Autodesk Inventor part; units mm, degrees
ref_plane "YZ Plane" through (0, 0, 0) normal (1, 0, 0) x (0, 1, 0)
ref_plane "XZ Plane" through (0, 0, 0) normal (0, 1, 0) x (-1, 0, 0)
ref_plane "XY Plane" through (0, 0, 0) normal (0, 0, 1) x (1, 0, 0)
sketch "Sketch2" plane through (0, 0, 1) normal (0, 0, 1) x (1, 0, 0)
  line L0 (-38.5, 36) -> (38.5, 36)
  line L1 (-48.5, 26) -> (-38.5, 26)
  line L2 (-38.5, 26) -> (-38.5, 36)
  line L3 (-38.5, 36) -> (-48.5, 36)
  line L4 (-48.5, 36) -> (-48.5, 26)
  line L5 (-48.5, 26) -> (-38.5, 36) construction
  line L6 (-38.5, 26) -> (-48.5, 36) construction
  line L7 (0, 0) -> (0, 7.0571)
  line L8 (0, 0) -> (6.6312, 0)
  line L9 (-38.5, -36) -> (-38.5, 36)
  line L10 (48.5, 26) -> (38.5, 26)
  line L11 (38.5, 26) -> (38.5, 36)
  line L12 (38.5, 36) -> (48.5, 36)
  line L13 (48.5, 36) -> (48.5, 26)
  line L14 (48.5, 26) -> (38.5, 36) construction
  line L15 (38.5, 26) -> (48.5, 36) construction
  circle A0 centre (-44.5, 31) radius 1.6
  circle A1 centre (44.5, 31) radius 1.6
  line L16 (38.5, -36) -> (-38.5, -36)
  line L17 (-5, -46) -> (5, -46)
  line L18 (5, -46) -> (5, -36)
  line L19 (5, -36) -> (-5, -36)
  line L20 (-5, -36) -> (-5, -46)
  line L21 (-5, -46) -> (5, -36) construction
  line L22 (5, -46) -> (-5, -36) construction
  circle A2 centre (0, -42) radius 1.6
  line L23 (-48.5, -26) -> (-38.5, -26)
  line L24 (-38.5, -26) -> (-38.5, -36)
  line L25 (-38.5, -36) -> (-48.5, -36)
  line L26 (-48.5, -36) -> (-48.5, -26)
  line L27 (-48.5, -26) -> (-38.5, -36) construction
  line L28 (-38.5, -26) -> (-48.5, -36) construction
  line L29 (38.5, -26) -> (38.5, -36)
  line L30 (38.5, -36) -> (48.5, -36)
  line L31 (48.5, -36) -> (48.5, -26)
  line L32 (48.5, -26) -> (38.5, -36) construction
  line L33 (38.5, -26) -> (48.5, -36) construction
  line L34 (48.5, -26) -> (38.5, -26)
  circle A3 centre (-44.5, -31) radius 1.6
  circle A4 centre (44.5, -31) radius 1.6
  point P0 (-43.5, 31)
  point P1 (43.5, 31)
  point P2 (0, -41)
  point P3 (-38.5, -36)
  point P4 (-43.5, -31)
  point P5 (43.5, -31)
  dimension "d5" = 10
  dimension "d6" = 10
  dimension "d10" = 3.2
  dimension "d12" = 4
  dimension "d18" = 3.2
  dimension "d19" = 10
  dimension "d20" = 10
  dimension "d21" = 4
  dimension "d22" = 5
sketch "Sketch1" plane through (0, 0, 0) normal (0, 0, 1) x (1, 0, 0)
  line L0 (-38.5, 36) -> (38.5, 36)
  line L1 (38.5, 36) -> (38.5, -36)
  line L2 (38.5, -36) -> (-38.5, -36)
  line L3 (-38.5, -36) -> (-38.5, 36)
  line L4 (-38.5, 36) -> (38.5, -36) construction
  line L5 (38.5, 36) -> (-38.5, -36) construction
  point P0 (0, 0)
  dimension "d0" = 72
  dimension "d1" = 77
extrude "Plate1" add sketch "Sketch1" along normal blind 1
sketch "Sketch3" plane through (0, 0, 1) normal (0, 0, 1) x (1, 0, 0)
  line L0 (-22.5, 27.5) -> (-12.5, 27.5)
  line L1 (-7.5, 22.5) -> (-7.5, 12.5)
  line L2 (-12.5, 7.5) -> (-22.5, 7.5)
  line L3 (-27.5, 12.5) -> (-27.5, 22.5)
  line L4 (-27.5, 27.5) -> (-7.5, 7.5) construction
  line L5 (-7.5, 27.5) -> (-27.5, 7.5) construction
  line L6 (-11.1923, 0) -> (11.1923, 0)
  line L7 (0, 8.4231) -> (0, -8.4231)
  arc A0 (-22.5, 27.5) -> (-27.5, 22.5) centre (-22.5, 22.5) ccw
  arc A1 (-7.5, 22.5) -> (-12.5, 27.5) centre (-12.5, 22.5) ccw
  arc A2 (-12.5, 7.5) -> (-7.5, 12.5) centre (-12.5, 12.5) ccw
  arc A3 (-27.5, 12.5) -> (-22.5, 7.5) centre (-22.5, 12.5) ccw
  line L8 (22.5, 27.5) -> (12.5, 27.5)
  line L9 (7.5, 22.5) -> (7.5, 12.5)
  line L10 (12.5, 7.5) -> (22.5, 7.5)
  line L11 (27.5, 12.5) -> (27.5, 22.5)
  line L12 (27.5, 27.5) -> (7.5, 7.5) construction
  line L13 (7.5, 27.5) -> (27.5, 7.5) construction
  arc A4 (27.5, 22.5) -> (22.5, 27.5) centre (22.5, 22.5) ccw
  arc A5 (12.5, 27.5) -> (7.5, 22.5) centre (12.5, 22.5) ccw
  arc A6 (7.5, 12.5) -> (12.5, 7.5) centre (12.5, 12.5) ccw
  arc A7 (22.5, 7.5) -> (27.5, 12.5) centre (22.5, 12.5) ccw
  line L14 (-22.5, -27.5) -> (-12.5, -27.5)
  line L15 (-7.5, -22.5) -> (-7.5, -12.5)
  line L16 (-12.5, -7.5) -> (-22.5, -7.5)
  line L17 (-27.5, -12.5) -> (-27.5, -22.5)
  line L18 (-27.5, -27.5) -> (-7.5, -7.5) construction
  line L19 (-7.5, -27.5) -> (-27.5, -7.5) construction
  arc A8 (-27.5, -22.5) -> (-22.5, -27.5) centre (-22.5, -22.5) ccw
  arc A9 (-12.5, -27.5) -> (-7.5, -22.5) centre (-12.5, -22.5) ccw
  arc A10 (-7.5, -12.5) -> (-12.5, -7.5) centre (-12.5, -12.5) ccw
  arc A11 (-22.5, -7.5) -> (-27.5, -12.5) centre (-22.5, -12.5) ccw
  line L20 (7.5, -22.5) -> (7.5, -12.5)
  arc A12 (12.5, -7.5) -> (7.5, -12.5) centre (12.5, -12.5) ccw
  arc A13 (7.5, -22.5) -> (12.5, -27.5) centre (12.5, -22.5) ccw
  line L21 (22.5, -27.5) -> (12.5, -27.5)
  line L22 (12.5, -7.5) -> (22.5, -7.5)
  line L23 (27.5, -27.5) -> (7.5, -7.5) construction
  line L24 (7.5, -27.5) -> (27.5, -7.5) construction
  arc A14 (27.5, -12.5) -> (22.5, -7.5) centre (22.5, -12.5) ccw
  line L25 (27.5, -12.5) -> (27.5, -22.5)
  arc A15 (22.5, -27.5) -> (27.5, -22.5) centre (22.5, -22.5) ccw
  point P0 (0, 0)
  point P1 (-17.5, 17.5)
  point P2 (0, 0)
  point P3 (17.5, 17.5)
  point P4 (-17.5, -17.5)
  point P5 (17.5, -17.5)
  dimension "d29" = 20
  dimension "d30" = 15
  dimension "d31" = 15
  dimension "d32" = 20
  dimension "d33" = 5
extrude "Cut1" cut sketch "Sketch3" against normal blind 1
sheet face with bend "Face2" sketch "Sketch2" thickness 1 toward (0, 0, -1) bend radius 1
bend "Bend1"
equation "\"d34\" = 厚度"
equation "\"d2\" = 厚度"
equation "\"d13\" = 折彎半徑"
equation "\"d14\" = 折彎離隙寬度"
equation "\"d16\" = 最小剩餘"
equation "\"d15\" = 折彎離隙深度"
equation "\"d17\" = 轉移半徑"
equation "\"折彎半徑\" = 厚度"
equation "\"折彎離隙寬度\" = 厚度"
equation "\"折彎離隙深度\" = 0.5 * 厚度"
equation "\"轉角離隙大小\" = 4 * 厚度"
equation "\"最小剩餘\" = 2 * 厚度"
equation "\"轉移半徑\" = 折彎半徑"
equation "\"Jacobi半徑大小\" = 折彎半徑"
equation "\"間隙大小\" = 厚度"
properties part number "battery_box_24V_top" material "Aluminum"
Source: CAD feature listing. Evaluate the final solid. Frame: model axes, mm. A direction names the side the tool comes from. Round coordinates to 2 decimals unless told otherwise and drop trailing zeros. Order: outer loops, then holes, each group sorted by start corner. A loop starts at its lowest first (then second) coordinate and runs counter-clockwise, first axis right, second up. Notation, with made-up numbers: (-11, 1) -> (24, 1) arc R15 ccw to (24, 18) -> close; hole circle Ø7 at (52, -23.5). An arc over 180 degrees is marked (long way). One line per item, written item: value. Start each with the question number.
Q1. Section query D-D (y = -42). Return the cut outline in (x, z), plus the area to 3 significant figures.
Q2. Access query for faces 3 (the flat face through (-1, 5, 1)), 4 (the cylindrical face through (8.93, -26, 0.51)). Directions: +Z, -Z, +X, -X, +Y, -Y. A direction counts if a zero-diameter tool reaches every point of the face in a straight line with its end or side. Return the directions, or none.
Q3. Section query B-B (x = 0). Return the cut outline in (y, z).
Q4. Material intervals for probe 1 along Y at (x, z) = (-44.5, 0.6); probe 2 along Y at (x, z) = (21, 0.1); probe 3 along X at (y, z) = (-15, 0.85), sorted ascending.
Q5. Section query C-C (x = -18). Return the cut outline in (y, z).
Q6. Draft query along Y for faces 1 (the cylindrical face through (-8.93, -9, 0.51)), 2 (the flat face through (-1, 5, 0)). Return one class per face: pulls with the +Y half, pulls with the -Y half, needs draft (parallel to the pull), parting line crosses it, or undercut.
Q7. Pin query (flat end, axial travel): pin 1 (0.5 mm diameter, centred on y = 19, z = 0.5, fed in from +X); pin 2 (0.5 mm diameter, centred on y = 12, z = 0.5, fed in from -X). Return the tip coordinate at first contact, or that it passes through.
Q8. Section query A-A (y = -31). Return the cut outline in (x, z).
Findings below:
1. outline: (-5, 0) -> (-1.6, 0) -> (-1.6, 1) -> (-5, 1) -> close; (1.6, 0) -> (5, 0) -> (5, 1) -> (1.6, 1) -> close
1. area: 6.80 mm²
2. face 3: +Z, +X, -X, +Y, -Y
2. face 4: +Z, -Z
3. outline: (-46, 0) -> (-43.6, 0) -> (-43.6, 1) -> (-46, 1) -> close; (-40.4, 0) -> (36, 0) -> (36, 1) -> (-40.4, 1) -> close
4. probe 1: -36 to -32.6, -29.4 to -26, 26 to 29.4, 32.6 to 36
4. probe 2: -36 to -27.5, -7.5 to 7.5, 27.5 to 36
4. probe 3: -38.5 to -27.5, -7.5 to 7.5, 27.5 to 38.5
5. outline: (-36, 0) -> (-27.5, 0) -> (-27.5, 1) -> (-36, 1) -> close; (-7.5, 0) -> (7.5, 0) -> (7.5, 1) -> (-7.5, 1) -> close; (27.5, 0) -> (36, 0) -> (36, 1) -> (27.5, 1) -> close
6. face 1: undercut
6. face 2: needs draft
7. pin 1: x = 38.5
7. pin 2: x = -38.5
8. outline: (-48.5, 0) -> (-46.1, 0) -> (-46.1, 1) -> (-48.5, 1) -> close; (-42.9, 0) -> (42.9, 0) -> (42.9, 1) -> (-42.9, 1) -> close; (46.1, 0) -> (48.5, 0) -> (48.5, 1) -> (46.1, 1) -> close
